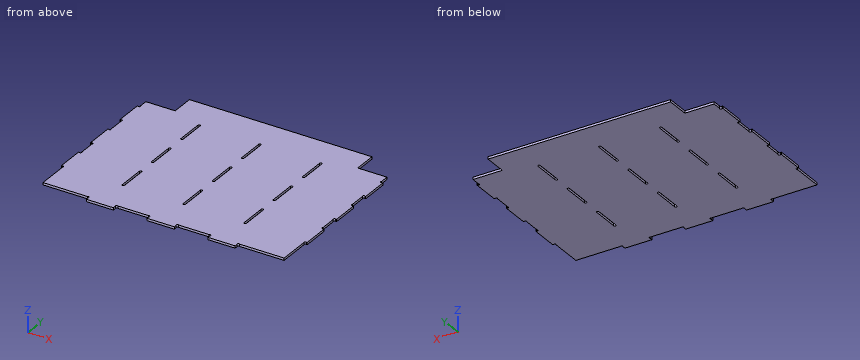
```python
from build123d import *

# Parameters (mm, degrees)
SKETCH1_W           = 338.325
SKETCH1_H           = 260.5
BOSS_EXTRUDE1_DEPTH = 1.5875
CUT_EXTRUDE1_DEPTH  = 3.175
SKETCH4_W           = 3.175
SKETCH4_H           = 38.1
SKETCH4_W_2         = 38.1
SKETCH4_H_2         = 6.35
BOSS_EXTRUDE2_DEPTH = 3.175
SKETCH5_R           = 1.5875
CUT_EXTRUDE3_DEPTH  = 3.175
SKETCH6_W           = 42.6875
SKETCH6_H           = 31.75
CUT_EXTRUDE4_DEPTH  = 3.175


with BuildPart() as part:
    # Sketch1 → Boss-Extrude1 (new body, symmetric)
    with BuildSketch(Plane.XY):
        with Locations((170.75, 133.425)):
            Rectangle(SKETCH1_W, SKETCH1_H)
    extrude(amount=BOSS_EXTRUDE1_DEPTH, both=True)

    # Sketch3 → Cut-Extrude1 (cut)
    with BuildSketch(Plane.XY.offset(1.5875)):
        with BuildLine():
            Line((169.1625, 217.6), (169.1625, 179.5))
            ThreePointArc((169.1625, 179.5), (170.75, 177.9125), (172.3375, 179.5))
            Line((172.3375, 179.5), (172.3375, 217.6))
            ThreePointArc((172.3375, 217.6), (170.75, 219.1875), (169.1625, 217.6))
        make_face()
        with BuildLine():
            Line((83.7875, 217.6), (83.7875, 179.5))
            ThreePointArc((83.7875, 179.5), (85.375, 177.9125), (86.9625, 179.5))
            Line((86.9625, 179.5), (86.9625, 217.6))
            ThreePointArc((86.9625, 217.6), (85.375, 219.1875), (83.7875, 217.6))
        make_face()
        with BuildLine():
            Line((254.5375, 217.6), (254.5375, 179.5))
            ThreePointArc((254.5375, 179.5), (256.125, 177.9125), (257.7125, 179.5))
            Line((257.7125, 179.5), (257.7125, 217.6))
            ThreePointArc((257.7125, 217.6), (256.125, 219.1875), (254.5375, 217.6))
        make_face()
        with BuildLine():
            Line((169.1625, 152.475), (169.1625, 114.375))
            ThreePointArc((169.1625, 114.375), (170.75, 112.7875), (172.3375, 114.375))
            Line((172.3375, 114.375), (172.3375, 152.475))
            ThreePointArc((172.3375, 152.475), (170.75, 154.0625), (169.1625, 152.475))
        make_face()
        with BuildLine():
            Line((83.7875, 152.475), (83.7875, 114.375))
            ThreePointArc((83.7875, 114.375), (85.375, 112.7875), (86.9625, 114.375))
            Line((86.9625, 114.375), (86.9625, 152.475))
            ThreePointArc((86.9625, 152.475), (85.375, 154.0625), (83.7875, 152.475))
        make_face()
        with BuildLine():
            Line((254.5375, 152.475), (254.5375, 114.375))
            ThreePointArc((254.5375, 114.375), (256.125, 112.7875), (257.7125, 114.375))
            Line((257.7125, 114.375), (257.7125, 152.475))
            ThreePointArc((257.7125, 152.475), (256.125, 154.0625), (254.5375, 152.475))
        make_face()
        with BuildLine():
            Line((169.1625, 87.35), (169.1625, 49.25))
            ThreePointArc((169.1625, 49.25), (170.75, 47.6625), (172.3375, 49.25))
            Line((172.3375, 49.25), (172.3375, 87.35))
            ThreePointArc((172.3375, 87.35), (170.75, 88.9375), (169.1625, 87.35))
        make_face()
        with BuildLine():
            Line((83.7875, 87.35), (83.7875, 49.25))
            ThreePointArc((83.7875, 49.25), (85.375, 47.6625), (86.9625, 49.25))
            Line((86.9625, 49.25), (86.9625, 87.35))
            ThreePointArc((86.9625, 87.35), (85.375, 88.9375), (83.7875, 87.35))
        make_face()
        with BuildLine():
            Line((254.5375, 87.35), (254.5375, 49.25))
            ThreePointArc((254.5375, 49.25), (256.125, 47.6625), (257.7125, 49.25))
            Line((257.7125, 49.25), (257.7125, 87.35))
            ThreePointArc((257.7125, 87.35), (256.125, 88.9375), (254.5375, 87.35))
        make_face()
    extrude(amount=-CUT_EXTRUDE1_DEPTH, mode=Mode.SUBTRACT)

    # Sketch4 → Boss-Extrude2 (add)
    with BuildSketch(Plane.XY.offset(1.5875)):
        with Locations((0, 198.55)):
            Rectangle(SKETCH4_W, SKETCH4_H)
        with Locations((0, 133.425)):
            Rectangle(SKETCH4_W, SKETCH4_H)
        with Locations((0, 68.3)):
            Rectangle(SKETCH4_W, SKETCH4_H)
        with Locations((85.375, 0)):
            Rectangle(SKETCH4_W_2, SKETCH4_H_2)
        with Locations((170.75, 0)):
            Rectangle(SKETCH4_W_2, SKETCH4_H_2)
        with Locations((256.125, 0)):
            Rectangle(SKETCH4_W_2, SKETCH4_H_2)
        with Locations((341.5, 68.3)):
            Rectangle(SKETCH4_W, SKETCH4_H)
        with Locations((341.5, 133.425)):
            Rectangle(SKETCH4_W, SKETCH4_H)
        with Locations((341.5, 198.55)):
            Rectangle(SKETCH4_W, SKETCH4_H)
    extrude(amount=-BOSS_EXTRUDE2_DEPTH)

    # Sketch5 → Cut-Extrude3 (cut)
    with BuildSketch(Plane.XY.offset(1.5875)):
        with Locations((0.464967985, 218.722532015)):
            Circle(SKETCH5_R)
        with Locations((0.464967985, 178.377467985)):
            Circle(SKETCH5_R)
        with Locations((0.464967985, 153.597532015)):
            Circle(SKETCH5_R)
        with Locations((0.464967985, 113.252467985)):
            Circle(SKETCH5_R)
        with Locations((0.464967985, 88.472532015)):
            Circle(SKETCH5_R)
        with Locations((0.464967985, 48.127467985)):
            Circle(SKETCH5_R)
        with Locations((341.035032015, 48.127467985)):
            Circle(SKETCH5_R)
        with Locations((341.035032015, 88.472532015)):
            Circle(SKETCH5_R)
        with Locations((341.035032015, 113.252467985)):
            Circle(SKETCH5_R)
        with Locations((341.035032015, 153.597532015)):
            Circle(SKETCH5_R)
        with Locations((341.035032015, 178.377467985)):
            Circle(SKETCH5_R)
        with Locations((341.035032015, 218.722532015)):
            Circle(SKETCH5_R)
        with Locations((65.202467985, 2.052467985)):
            Circle(SKETCH5_R)
        with Locations((105.547532015, 2.052467985)):
            Circle(SKETCH5_R)
        with Locations((150.577467985, 2.052467985)):
            Circle(SKETCH5_R)
        with Locations((190.922532015, 2.052467985)):
            Circle(SKETCH5_R)
        with Locations((235.952467985, 2.052467985)):
            Circle(SKETCH5_R)
        with Locations((276.297532015, 2.052467985)):
            Circle(SKETCH5_R)
    extrude(amount=-CUT_EXTRUDE3_DEPTH, mode=Mode.SUBTRACT)

    # Sketch6 → Cut-Extrude4 (cut)
    with BuildSketch(Plane.XY.offset(1.5875)):
        with Locations((320.15625, 247.8)):
            Rectangle(SKETCH6_W, SKETCH6_H)
        with Locations((21.34375, 247.8)):
            Rectangle(SKETCH6_W, SKETCH6_H)
    extrude(amount=-CUT_EXTRUDE4_DEPTH, mode=Mode.SUBTRACT)


solid = part.part
```
Can you work these out from the model? Positions are in its coordinate system, mm. Give positions to 0.01 mm unless a question says otherwise; leave off trailing zeros. Loops run counter-clockwise (first coordinate to the right, second up) from the corner with the lowest first, then second, coordinate; pieces in that order, holes last. Notation, with made-up numbers: M 10,45.25 L 69,45.25 A24 ccw 69,73.25 Z; hole C 40,5 d2. An arc over 180 degrees is marked long. One line per question, with ' | ' between items. Start each with the question number.
Q1. If we section it at B-B (z = -1): State how many separate pieces and enclosed holes the cut face has, plus the area to 3 significant figures.
Q2. If we section it at A-A (y = 188): Please give me the cut outline in (x, z), plus the area to 3 significant figures.
Q3. If we section it at C-C (x = 127): Please give me the cut outline in (y, z) (1 decimal), plus the area to 3 significant figures.
Q4. For pin 1 Ø1 at (x, z) = (-1, -0.5) entering from -Y; pin 2 Ø1 at (x, z) = (137, 0) entering from -Y (3 decimals); pin 3 Ø0.7 at (x, z) = (-1, 0.5) entering from +Y, each with a flat end and sliding along its axis, tell me the tip position at first contact or that it passes through.
Q5. If we section it at D-D (y = 98.5): Please give me the cut outline in (x, z).
Q6. If I drill on line 1 (X direction, y = 203.5, z = -0.45); line 2 (X direction, y = 178.5, z = 1.45); line 3 (X direction, y = 91, z = 0.75), over which ranges is the centre line in solid material (lowest first)? Write a range as from..to.
Computed:
1) separate pieces: 1 | enclosed holes: 9 | area: 85,800 mm²
2) outline: M -1.59,-1.59 L 83.79,-1.59 L 83.79,1.59 L -1.59,1.59 Z; M 86.96,-1.59 L 169.16,-1.59 L 169.16,1.59 L 86.96,1.59 Z; M 172.34,-1.59 L 254.54,-1.59 L 254.54,1.59 L 172.34,1.59 Z; M 257.71,-1.59 L 343.09,-1.59 L 343.09,1.59 L 257.71,1.59 Z | area: 1,060 mm²
3) outline: M 3.2,-1.6 L 263.7,-1.6 L 263.7,1.6 L 3.2,1.6 Z | area: 827 mm²
4) pin 1: stops at y = 49.25 | pin 2: stops at y = 3.175 | pin 3: stops at y = 217.6
5) outline: M 1.59,-1.59 L 339.91,-1.59 L 339.91,1.59 L 1.59,1.59 Z
6) line 1: x = -1.59..83.79, 86.96..169.16, 172.34..254.54, 257.71..343.09 | line 2: x = 2.05..84.14, 86.61..169.52, 171.98..254.89, 257.36..339.45 | line 3: x = 1.59..339.91
